from build123d import *

# Parameters (mm, degrees)
SKETCH1_R           = 4.7625
BOSS_EXTRUDE1_DEPTH = 25.4
SKETCH2_R           = 3.9751
BOSS_EXTRUDE2_DEPTH = 7.366
SKETCH3_R           = 2.38125
CUT_EXTRUDE1_DEPTH  = 33.766
SKETCH4_R           = 3.4544
CUT_EXTRUDE2_DEPTH  = 12.7


with BuildPart() as part:
    # Sketch1 → Boss-Extrude1 (new body)
    with BuildSketch(Plane(origin=(0, 0, 0), x_dir=(1, 0, 0), z_dir=(0, 1, 0))):
        with Locations(Location((0, 0, 0), (0, 0, 270))):  # turned: the seam where the file's is
            Circle(SKETCH1_R)
    extrude(amount=BOSS_EXTRUDE1_DEPTH)

    # Sketch2 → Boss-Extrude2 (add)
    with BuildSketch(Plane(origin=(0, 25.4, 0), x_dir=(1, 0, 0), z_dir=(0, 1, 0))):
        with Locations(Location((0, 0, 0), (0, 0, 270))):  # turned: the seam where the file's is
            Circle(SKETCH2_R)
    extrude(amount=BOSS_EXTRUDE2_DEPTH)

    # Sketch3 → Cut-Extrude1 (cut, through all)
    with BuildSketch(Plane.XZ):
        with Locations(Location((0, 0, 0), (0, 0, 270))):  # turned: the seam where the file's is
            Circle(SKETCH3_R)
    extrude(amount=-CUT_EXTRUDE1_DEPTH, mode=Mode.SUBTRACT)

    # Sketch4 → Cut-Extrude2 (cut)
    with BuildSketch(Plane.XZ):
        with Locations(Location((0, 0, 0), (0, 0, 270))):  # turned: the seam where the file's is
            Circle(SKETCH4_R)
    extrude(amount=-CUT_EXTRUDE2_DEPTH, mode=Mode.SUBTRACT)


solid = part.part
Part model, mm, in its own coordinate system. Coordinates: 2 decimals unless noted, no trailing zeros. Order: outer loops, then holes, each group sorted by start corner. A loop starts at its lowest first (then second) coordinate and runs counter-clockwise, first axis right, second up. Notation, with made-up numbers: (-20, 24.5) - (33, 24.5) arc R28 ccw to (33, 51.5) - close; hole circle Ø8 at (-4, 88). An arc over 180 degrees is marked (long way). Use CSV: the item, a comma, the result in double quotes.
Item 1: Drop flat-ended pins along their axis: P1, Ø1.5, axis at x = -2.5, y = 7.5, coming from the -Z side; P2, Ø5, axis at y = 10.5, z = -3.5, coming from the +X side; P3, Ø1.5, axis at x = -2.5, y = 18, coming from the +Z side. Give the stop position or say it passes through.
Solved:
P1,"stops at z = -4.43"
P2,"stops at x = 4.66"
P3,"stops at z = 4.43"
Item 2: Saw through at B-B on z = 0. Give the cut face in (x, y).
Solved:
outline,"(-4.76, 0) - (-3.45, 0) - (-3.45, 12.7) - (-2.38, 12.7) - (-2.38, 32.77) - (-3.98, 32.77) - (-3.98, 25.4) - (-4.76, 25.4) - close; (2.38, 12.7) - (3.45, 12.7) - (3.45, 0) - (4.76, 0) - (4.76, 25.4) - (3.98, 25.4) - (3.98, 32.77) - (2.38, 32.77) - close"
Item 3: Saw through at D-D on z = 3. Give the cut face in (x, y).
Solved:
outline,"(-3.7, 0) - (-1.71, 0) - (-1.71, 12.7) - (1.71, 12.7) - (1.71, 0) - (3.7, 0) - (3.7, 25.4) - (2.61, 25.4) - (2.61, 32.77) - (-2.61, 32.77) - (-2.61, 25.4) - (-3.7, 25.4) - close"
Item 4: Mould opens along X. For faces 1 (the face through (-3, 25.4, -3)), 2 (the face through (-3.37, 6.26, 0.75)), 3 (the face through (-3.53, 29.03, 1.83)) say: +X half, -X half, draft (parallel to the pull), parting line (faces both ways), or undercut.
Solved:
face 1,"draft"
face 2,"undercut"
face 3,"parting line"
Item 5: Saw through at C-C on y = 27.5. Give the cut face in (x, z).
Solved:
outline,"circle Ø7.95 at (0, 0); hole circle Ø4.76 at (0, 0)"
Item 6: Probe probe 1 along X at (y, z) = (5.75, 0); probe 2 along X at (y, z) = (18, 0); probe 3 along Y at (x, z) = (2, -2). List the from-to ranges inside material, lowest first.
Solved:
probe 1,"x = -4.76 to -3.45, 3.45 to 4.76"
probe 2,"x = -4.76 to -2.38, 2.38 to 4.76"
probe 3,"y = 12.7 to 32.77"
Item 7: Saw through at A-A on x = 0. Give the cut face in (y, z).
Solved:
outline,"(0, -4.76) - (25.4, -4.76) - (25.4, -3.98) - (32.77, -3.98) - (32.77, -2.38) - (12.7, -2.38) - (12.7, -3.45) - (0, -3.45) - close; (0, 3.45) - (12.7, 3.45) - (12.7, 2.38) - (32.77, 2.38) - (32.77, 3.98) - (25.4, 3.98) - (25.4, 4.76) - (0, 4.76) - close"
